```python
from build123d import *

# Parameters (mm, degrees)
SKETCH010_W     = 99.15
SKETCH010_H     = 28
PAD005_DEPTH    = 3.6
SKETCH011_R     = 3
SKETCH011_R_2   = 1.1
PAD006_DEPTH    = 2
SKETCH015_R     = 1
POCKET002_DEPTH = 5


with BuildPart() as part:
    # Sketch010 → Pad005 (new body)
    with BuildSketch(Plane.XY):
        with BuildLine():
            Line((0, -3), (109.15, -3))
            ThreePointArc((109.15, -3), (111.27132, -2.12132), (112.15, 0))
            Line((112.15, 0), (112.15, 28))
            ThreePointArc((112.15, 28), (111.27132, 30.12132), (109.15, 31))
            Line((109.15, 31), (0, 31))
            ThreePointArc((0, 31), (-2.12132, 30.12132), (-3, 28))
            Line((-3, 28), (-3, 0))
            ThreePointArc((-3, 0), (-2.12132, -2.12132), (0, -3))
        make_face()
        with Locations((54.575, 14)):
            Rectangle(SKETCH010_W, SKETCH010_H, mode=Mode.SUBTRACT)
    extrude(amount=PAD005_DEPTH)

    # Sketch011 → Pad006 (join)
    with BuildSketch(Plane.XY):
        with Locations((75.675, 25.83)):
            Circle(SKETCH011_R)
        with Locations((75.675, 25.83)):
            Circle(SKETCH011_R_2, mode=Mode.SUBTRACT)
        with Locations((75.675, 2.5746)):
            Circle(SKETCH011_R)
        with Locations((75.675, 2.5746)):
            Circle(SKETCH011_R_2, mode=Mode.SUBTRACT)
        with Locations((7.73, 20.36)):
            Circle(SKETCH011_R)
        with Locations((7.73, 20.36)):
            Circle(SKETCH011_R_2, mode=Mode.SUBTRACT)
    extrude(amount=PAD006_DEPTH)

    # Sketch015 → Pocket002 (cut)
    with BuildSketch(Plane.XY.offset(2)):
        with Locations((5, 28)):
            Circle(SKETCH015_R)
        with Locations((104.15, 28)):
            Circle(SKETCH015_R)
        with Locations((104.15, 0)):
            Circle(SKETCH015_R)
        with Locations((5, 0)):
            Circle(SKETCH015_R)
    extrude(amount=POCKET002_DEPTH, mode=Mode.SUBTRACT)


solid = part.part
```
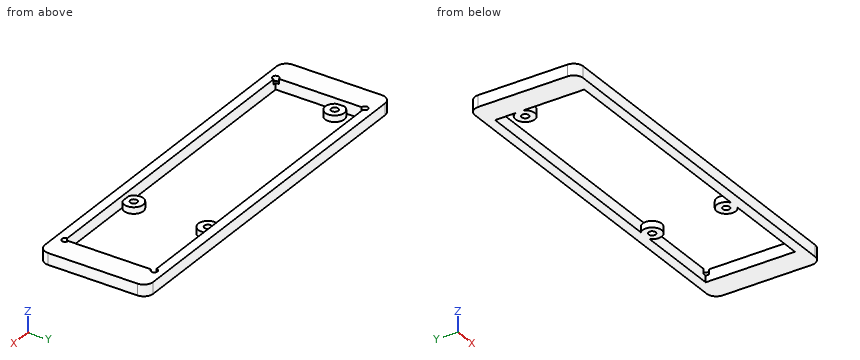
Can you work these out from the model? Positions are in its coordinate system, mm. Give positions to 0.01 mm unless a question says otherwise; leave off trailing zeros. Loops run counter-clockwise (first coordinate to the right, second up) from the corner with the lowest first, then second, coordinate; pieces in that order, holes last. Notation, with made-up numbers: M 70.5,60 L 127.5,60 A28 ccw 127.5,99 Z; hole C 42.5,-33.5 d1. An arc over 180 degrees is marked long. Use one line per item in the form item = value. Start each with the question number.
(1) I want a section at B-B, the plane z = 2.6. Write out the boundary of the cut face in (x, y).
(2) I want a section at D-D, the plane x = 7.73. Write out the boundary of the cut face in (y, z), and give its area (3 significant figures).
(3) Please list where these lines run through material, in increasing order: line 1 (X direction, y = 2.5, z = 0.5); line 2 (X direction, y = 11.5, z = 2.9); line 3 (Y direction, x = 42.5, z = 3.25).
(4) I want a section at C-C, the plane y = 20.36. Write out the boundary of the cut face in (x, z), and give its area (3 significant figures).
(5) I want a section at A-A, the plane y = 8.5. Write out the boundary of the cut face in (x, z), and give its area (3 significant figures).
(6) I'm going to push flat-ended pins straight in: P1, Ø1, axis at x = 5, y = 0, coming from the +Z side; P2, Ø2, axis at x = 75.68, y = 2.57, coming from the -Z side. Where does each tip first touch, or does it pass through?
Worked out:
q1.outline = M -3,0 A3 ccw 0,-3 L 109.15,-3 A3 ccw 112.15,0 L 112.15,28 A3 ccw 109.15,31 L 0,31 A3 ccw -3,28 Z; hole M 5,1 A1 ccw long 6,0 L 103.15,0 A1 ccw long 104.15,1 L 104.15,27 A1 ccw long 103.15,28 L 6,28 A1 ccw long 5,27 Z
q2.outline = M -3,0 L 0,0 L 0,3.6 L -3,3.6 Z; M 17.36,0 L 19.26,0 L 19.26,2 L 17.36,2 Z; M 21.46,0 L 23.36,0 L 23.36,2 L 21.46,2 Z; M 28,0 L 31,0 L 31,3.6 L 28,3.6 Z
q2.area = 29.2 mm²
q3.line_1 = -3 to 5, 72.68 to 74.58, 76.77 to 78.67, 104.15 to 112.15
q3.line_2 = -3 to 5, 104.15 to 112.15
q3.line_3 = -3 to 0, 28 to 31
q4.outline = M -3,0 L 6.63,0 L 6.63,2 L 5,2 L 5,3.6 L -3,3.6 Z; M 8.83,0 L 10.73,0 L 10.73,2 L 8.83,2 Z; M 104.15,0 L 112.15,0 L 112.15,3.6 L 104.15,3.6 Z
q4.area = 64.7 mm²
q5.outline = M -3,0 L 5,0 L 5,3.6 L -3,3.6 Z; M 104.15,0 L 112.15,0 L 112.15,3.6 L 104.15,3.6 Z
q5.area = 57.6 mm²
q6.P1 = 2
q6.P2 = through
